Could you check a few things on this model? Use its own coordinates, in mm. Round coordinates to 2 decimals unless told otherwise and drop trailing zeros. Write each loop counter-clockwise with the first axis right and the second up, starting at its lowest first coordinate (ties: lowest second). Pieces come first, ordered by that corner, then holes. Notation, with made-up numbers: (43.25, 77.25) -> (89.25, 77.25) arc R34 ccw to (89.25, 110.25) -> close; hole circle Ø11 at (-29, 29.5). An arc over 180 degrees is marked (long way). Return JSON: item names as keys, results as strings.
from build123d import *
from build123d.topology import SkipClean

# Parameters (mm, degrees)
BASPROSKE_W                 = 20
BASPROSKE_H                 = 9
TOOTHCUT_DEPTH              = 24.706539182
TEETHCUTS_COUNT             = 10
TEETHCUTS_ANGLE             = 324
BORSKE_R                    = 2.5
BORE_DEPTH                  = 50.0000508
IZIM1_R                     = 3
Y_KSEKLIK_EKSTR_ZYON3_DEPTH = 20
Y_KSEKLIK_EKSTR_ZYON4_START = 15
IZIM2_R                     = 9
Y_KSEKLIK_EKSTR_ZYON4_DEPTH = 15


with BuildPart() as part:
    # BasProSke → Base-Revolve (revolve)
    with BuildSketch(Plane(origin=(0, 0, 0), x_dir=(1, 0, 0), z_dir=(0, 1, 0)), mode=Mode.PRIVATE) as base_revolve_sk:
        with Locations((10, 4.5)):
            Rectangle(BASPROSKE_W, BASPROSKE_H)
    revolve(base_revolve_sk.sketch.rotate(Axis((-10, 0, 0), (1, 0, 0)), 180), axis=Axis((-10, 0, 0), (1, 0, 0)))

    # TooCutSke → ToothCut (cut, through all)
    with BuildSketch(Plane(origin=(0, 0, 0), x_dir=(0, 0, -1), z_dir=(1, 0, 0))):
        with BuildLine():
            ThreePointArc((0.883878355, 5.554109745), (0, 5.624), (-0.883878355, 5.554109745))
            ThreePointArc((-0.883878355, 5.554109745), (-1.258245767, 7.379188248), (-2.637816971, 8.631324741))
            ThreePointArc((-2.637816971, 8.631324741), (0, 9.0254), (2.637816971, 8.631324741))
            ThreePointArc((2.637816971, 8.631324741), (1.258245767, 7.379188248), (0.883878355, 5.554109745))
        make_face()
    toothcut = extrude(amount=TOOTHCUT_DEPTH, mode=Mode.SUBTRACT)

    # TeethCuts: ToothCut ×10 about axis
    teethcuts_axis = Axis((-10, 0, 0), (1, 0, 0))
    for i in range(1, TEETHCUTS_COUNT):
        add(toothcut.rotate(teethcuts_axis, i * TEETHCUTS_ANGLE / (TEETHCUTS_COUNT - 1)), mode=Mode.SUBTRACT)

    # BorSke → Bore (cut, symmetric)
    with BuildSketch(Plane(origin=(0, 0, 0), x_dir=(0, 0, -1), z_dir=(1, 0, 0))):
        with Locations(Location((0, 0, 0), (0, 0, 180))):
            Circle(BORSKE_R)
    extrude(amount=BORE_DEPTH, both=True, mode=Mode.SUBTRACT)

    # Çizim1 → Yükseklik-Ekstrüzyon3 (add)
    with BuildSketch(Plane(origin=(20, 0, 0), x_dir=(0, 0, -1), z_dir=(1, 0, 0))):
        Circle(IZIM1_R)
    extrude(amount=-Y_KSEKLIK_EKSTR_ZYON3_DEPTH)

    # Çizim2 → Yükseklik-Ekstrüzyon4 (add)
    with SkipClean():  # the faces are left unmerged after this step: merging them gives an invalid solid
        with BuildSketch(Plane(origin=(20, 0, 0), x_dir=(0, 0, -1), z_dir=(1, 0, 0)).offset(Y_KSEKLIK_EKSTR_ZYON4_START)):
            with Locations(Location((0, 0, 0), (0, 0, 178.810548778))):
                Circle(IZIM2_R)
        extrude(amount=-Y_KSEKLIK_EKSTR_ZYON4_DEPTH)


solid = part.part
1) If I drill on probe 1 along Y at (x, z) = (4, -6.5); probe 2 along Z at (x, y) = (13.5, 4.5); probe 3 along Y at (x, z) = (14, 6.75), over which ranges is the centre line in solid material (lowest first)? Write a range as [from, to].
Return value:
{"probe 1": "[-5.5, -3.34], [-1.13, 1.13], [3.34, 5.5]", "probe 2": "[-7.24, -4.36], [-3.37, 3.37], [4.36, 7.24]", "probe 3": "[-5.49, -3.62], [-1.15, 1.15], [3.62, 5.49]"}
2) I want a section at C-C, the plane x = 23.5. Please give me the cut outline in (y, z).
Return value:
{"outline": "circle Ø18 at (0, 0)"}
3) I want a section at A-A, the plane z = 0. Please give me the cut outline in (x, y), and give its area (3 significant figures).
Return value:
{"outline": "(0, -5.62) -> (20, -5.62) -> (20, -9) -> (35, -9) -> (35, 9) -> (20, 9) -> (20, 5.62) -> (0, 5.62) -> close", "area": "495 mm²"}
4) Will these pins go through, and if not, where does the flat tip stop? pin 1 Ø10 at (x, z) = (6, -5.5) entering from -Y; pin 2 Ø1.5 at (x, z) = (27.5, 2) entering from -Y; pin 3 Ø1.2 at (y, z) = (-2, -8) entering from -X.
Return value:
{"pin 1": "y = -8.62", "pin 2": "y = -8.91", "pin 3": "x = 20"}
5) I want a section at D-D, the plane y = 3.5. Please give me the cut outline in (x, z), and give its area (3 significant figures).
Return value:
{"outline": "(0, -6.65) -> (20, -6.65) -> (20, -8.29) -> (35, -8.29) -> (35, 8.29) -> (20, 8.29) -> (20, 6.65) -> (0, 6.65) -> close", "area": "515 mm²"}
6) Thinking about a two-plate mould opening in Y: for faces 1 (the face through (20, -2, 7)), 2 (the face through (35, 0, 0)), which applies, pulls with the +Y half, pulls with the -Y half, needs draft (parallel to the pull), parting line crosses it, or undercut?
Return value:
{"face 1": "undercut", "face 2": "needs draft"}
7) I want a section at B-B, the plane y = -6.5. Please give me the cut outline in (x, z), and give its area (3 significant figures).
Return value:
{"outline": "(0, -3.29) -> (20, -3.29) -> (20, -6.22) -> (35, -6.22) -> (35, 6.22) -> (20, 6.22) -> (20, 3.29) -> (0, 3.29) -> (0, 0.93) -> (20, 0.93) -> (20, -0.93) -> (0, -0.93) -> close", "area": "281 mm²"}
